Solid Edge part; units mm, degrees
sketch "Sketch1" plane through (0, 0, 0) normal (0, 0, 1) x (1, 0, 0)
  circle A0 centre (0, 0) radius 3
  circle A1 centre (0, 0) radius 9.5
extrude "Protrusion1" add sketch "Sketch1" along normal mid plane 6
sketch "Sketch2" plane through (0, 0, 0) normal (0, -1, 0) x (1, 0, 0)
  line L0 (7.6295, 2.5394) -> (7.6295, 3.4504)
  line L1 (6.263, 2.5394) -> (7.6295, 2.5394)
  line L2 (6.263, 2.5394) -> (5.1623, 2.5394)
  line L3 (5.1623, 2.5394) -> (5.1623, 3.4504)
revolve "RevolvedCutout1" cut sketch "Sketch2" angle 360 about axis through (0, 0, -54) along (0, 0, 1) material side at (7.5795, 0, 2.9949)
mirror "Mirror1" about plane through (0, 0, 0) normal (0, 0, 1) of "RevolvedCutout1"
CAD build for the part. Positions are in the model's coordinates, mm. A direction names the side the tool comes from. Give positions to 0.01 mm unless a question says otherwise; leave off trailing zeros. Order: outer loops, then holes, each group sorted by start corner. A loop starts at its lowest first (then second) coordinate and runs counter-clockwise, first axis right, second up.
(1) Tool access for faces 1 (the flat face through (2, -5, 2.539)), 2 (the flat face through (-2, -5, -2.539)), 3 (the cylindrical face through (-3, 0, 0)): list every direction of +Z, -Z, +X, -X, +Y, -Y with a clear straight run to the whole face (end or side of a thin tool).
(2) Saw through at A-A, the plane y = 0. Give the cut face in (x, z), then the cut area to 3 significant figures.
(3) Drill centre lines: L1, parallel to Y at x = 0, z = -2.7; L2, parallel to X at y = 2.25, z = 0.9; L3, parallel to Z at x = 1.5, y = 6.25. Where is each one in solid material? Low to high.
(4) Saw through at C-C, the plane y = -7. Give the cut face in (x, z), then the cut area to 3 significant figures.
(5) Flat gauge pins, fed straight in: pin 1 (2 mm diameter, centred on x = -5.5, z = -2, fed in from -Y); pin 2 (3 mm diameter, centred on y = -2, z = 0, fed in from +X); pin 3 (1 mm diameter, centred on y = -2.5, z = 0.5, fed in from -X). Where does each tip first touch, or does it go through?
(6) Saw through at D-D, the plane x = -4. Give the cut face in (y, z), then the cut area to 3 significant figures.
(7) Mould opens along X. For faces 4 (the flat face through (0, 8, -3)), 5 (the cylindrical face through (4.38, 8.43, -0.04)), 6 (the cylindrical face through (-3.805, 3.489, 2.773)) say: released by +X, released by -X, zero draft, split by the parting line, or undercut.
Results found:
1. face 1: +Z
1. face 2: -Z
1. face 3: +Z, -Z
2. outline: (-9.5, -3) - (-7.63, -3) - (-7.63, -2.54) - (-5.16, -2.54) - (-5.16, -3) - (-3, -3) - (-3, 3) - (-5.16, 3) - (-5.16, 2.54) - (-7.63, 2.54) - (-7.63, 3) - (-9.5, 3) - close; (3, -3) - (5.16, -3) - (5.16, -2.54) - (7.63, -2.54) - (7.63, -3) - (9.5, -3) - (9.5, 3) - (7.63, 3) - (7.63, 2.54) - (5.16, 2.54) - (5.16, 3) - (3, 3) - close
2. area: 73.5 mm2
3. L1: y = -9.5 to -7.63, -5.16 to -3, 3 to 5.16, 7.63 to 9.5
3. L2: x = -9.23 to -1.98, 1.98 to 9.23
3. L3: z = -2.54 to 2.54
4. outline: (-6.42, -3) - (-3.03, -3) - (-3.03, -2.54) - (3.03, -2.54) - (3.03, -3) - (6.42, -3) - (6.42, 3) - (3.03, 3) - (3.03, 2.54) - (-3.03, 2.54) - (-3.03, 3) - (-6.42, 3) - close
4. area: 71.5 mm2
5. pin 1: stops at y = -8.37
5. pin 2: stops at x = 9.49
5. pin 3: stops at x = -9.29
6. outline: (-8.62, -3) - (-6.5, -3) - (-6.5, -2.54) - (-3.26, -2.54) - (-3.26, -3) - (3.26, -3) - (3.26, -2.54) - (6.5, -2.54) - (6.5, -3) - (8.62, -3) - (8.62, 3) - (6.5, 3) - (6.5, 2.54) - (3.26, 2.54) - (3.26, 3) - (-3.26, 3) - (-3.26, 2.54) - (-6.5, 2.54) - (-6.5, 3) - (-8.62, 3) - close
6. area: 97.4 mm2
7. face 4: zero draft
7. face 5: split by the parting line
7. face 6: undercut
